Could you check a few things on this drawing? It's one solid part, dimensions in mm from its lowest x, y, z. Give positions to 0.01 mm unless a question says otherwise; leave off trailing zeros. Loops run counter-clockwise (first coordinate to the right, second up) from the corner with the lowest first, then second, coordinate; pieces in that order, holes last. Notation, with made-up numbers: (29.5, 50) -> (41.5, 50) arc R19 cw to (41.5, 81) -> close; hole circle Ø3 at (35.25, 52.25). An arc over 180 degrees is marked (long way). Use CSV: the item, a comma, the result in double quotes.
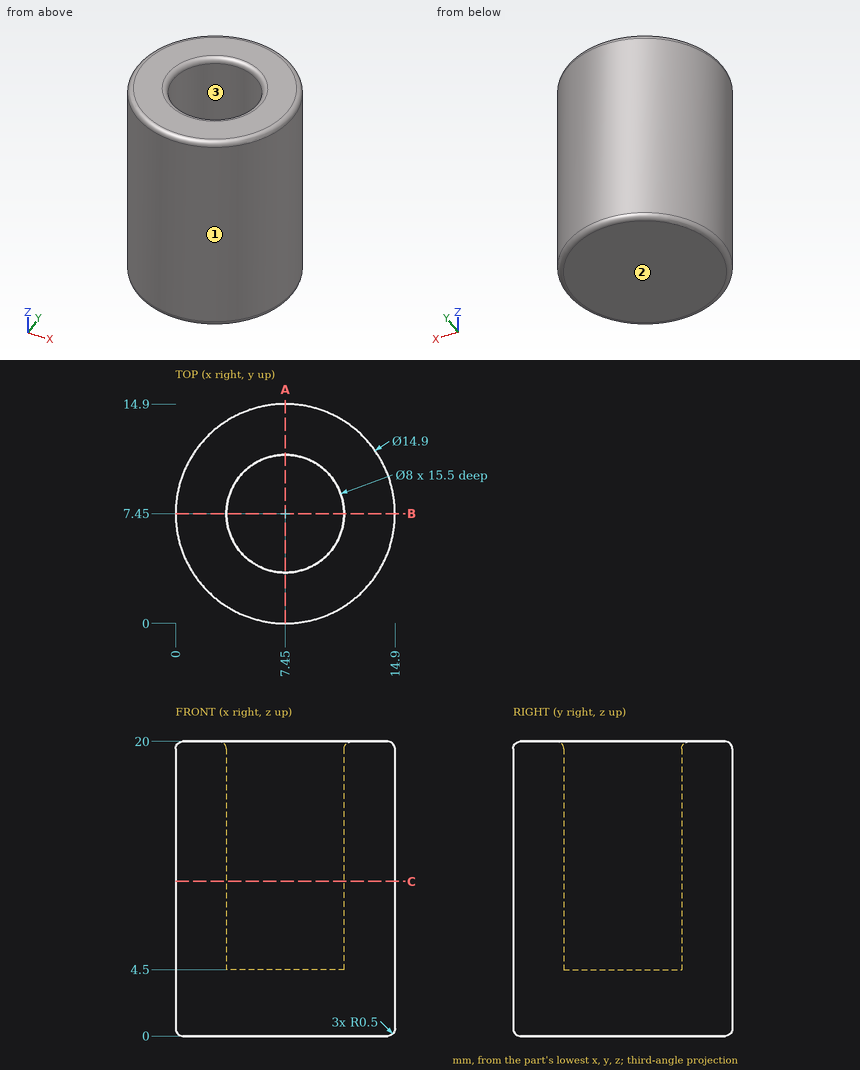
(1) We'd pull the mould along Y, two halves only. Please class the marked faces 1, 2 and 3: released by +Y, released by -Y, zero draft, split by the parting line, or undercut.
Answer sheet:
face 1,"split by the parting line"
face 2,"zero draft"
face 3,"undercut"
(2) If I drill on L1, parallel to Y at x = 7.45, z = 10.25; L2, parallel to Z at x = 6.75, y = 10.75; L3, parallel to Y at x = 8.5, z = 7.75, over which ranges is the centre line in solid material (lowest first)? Write a range as from..to.
Answer sheet:
L1,"y = 0..3.45, 11.45..14.9"
L2,"z = 0..4.5"
L3,"y = 0.07..3.59, 11.31..14.83"
(3) Will these pins go through, and if not, where does the flat tip stop? pin 1 Ø8 at (x, y) = (7.5, 10.5) entering from +Z; pin 2 Ø2 at (y, z) = (12.5, 17) entering from +X; pin 3 Ø8 at (x, z) = (12, 2.5) entering from -Y; pin 4 Ø4 at (x, y) = (7, 6.5) entering from +Z.
Answer sheet:
pin 1,"stops at z = 20"
pin 2,"stops at x = 13.7"
pin 3,"stops at y = 0.02"
pin 4,"stops at z = 4.5"
(4) If we section it at A-A, the plane x = 7.45: Write out the boundary of the cut face in (y, z).
Answer sheet:
outline,"(0, 0.5) arc R0.5 ccw to (0.5, 0) -> (14.4, 0) arc R0.5 ccw to (14.9, 0.5) -> (14.9, 19.5) arc R0.5 ccw to (14.4, 20) -> (11.95, 20) arc R0.5 ccw to (11.45, 19.5) -> (11.45, 4.5) -> (3.45, 4.5) -> (3.45, 19.5) arc R0.5 ccw to (2.95, 20) -> (0.5, 20) arc R0.5 ccw to (0, 19.5) -> close"
(5) If we section it at C-C, the plane z = 10.5: Write out the boundary of the cut face in (x, y), then the cut area to 3 significant figures.
Answer sheet:
outline,"circle Ø14.9 at (7.45, 7.45); hole circle Ø8 at (7.45, 7.45)"
area,"124 mm2"
